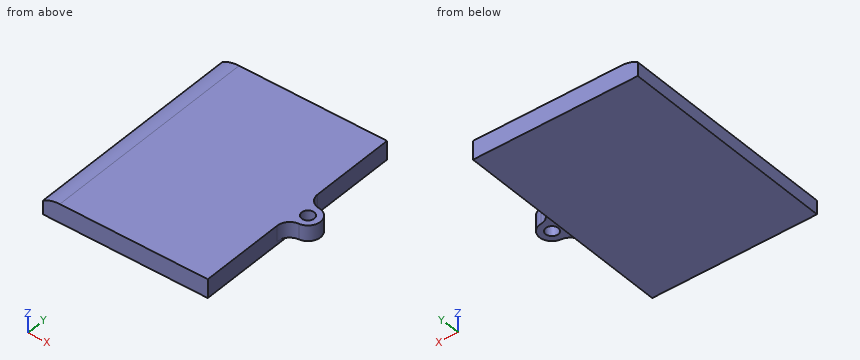
from build123d import *

# Parameters (mm, degrees)
BOSS_EXTRUDE1_DEPTH = 35.4
SKETCH2_W           = 28.62824493
SKETCH2_H           = 44.507069041
CUT_EXTRUDE1_DEPTH  = 36
SKETCH3_W           = 27
SKETCH3_H           = 2
CUT_EXTRUDE2_DEPTH  = 39.528041736
SKETCH4_W           = 4.666859097
SKETCH4_H           = 39.875061907
SKETCH4_W_2         = 6.439084071
SKETCH4_H_2         = 41.174693554
CUT_EXTRUDE3_DEPTH  = 39.563713514
SKETCH5_R           = 1
BOSS_EXTRUDE2_DEPTH = 2.5
FILLET1_R           = 2


with BuildPart() as part:
    # Sketch1 → Boss-Extrude1 (new body)
    with BuildSketch(Plane(origin=(0, 0, 0), x_dir=(1, 0, 0), z_dir=(0, 1, 0))):
        with BuildLine():
            Line((-17, 2.5), (-12, 2.5))
            Line((-12, 2.5), (12, 2.5))
            Line((12, 2.5), (12, -2.5))
            Line((12, -2.5), (-12, -2.5))
            ThreePointArc((-12, -2.5), (-15.535533906, -1.035533906), (-17, 2.5))
        make_face()
    extrude(amount=BOSS_EXTRUDE1_DEPTH)

    # Sketch2 → Cut-Extrude1 (cut)
    with BuildSketch(Plane(origin=(0, 0, -2.5), x_dir=(-1, 0, 0), z_dir=(0, 0, -1))):
        with Locations((29.314122465, 17.150131431)):
            Rectangle(SKETCH2_W, SKETCH2_H)
    extrude(amount=-CUT_EXTRUDE1_DEPTH, mode=Mode.SUBTRACT)

    # Sketch3 → Cut-Extrude2 (cut, through all)
    with BuildSketch(Plane(origin=(0, 35.4, 0), x_dir=(1, 0, 0), z_dir=(0, 1, 0))):
        with Locations((-1.5, 1.5)):
            Rectangle(SKETCH3_W, SKETCH3_H)
    extrude(amount=-CUT_EXTRUDE2_DEPTH, mode=Mode.SUBTRACT)

    # Sketch4 → Cut-Extrude3 (cut, through all)
    with BuildSketch(Plane(origin=(0, 0, -0.5), x_dir=(-1, 0, 0), z_dir=(0, 0, -1))):
        with Locations((-14.033429549, 18.67919463)):
            Rectangle(SKETCH4_W, SKETCH4_H)
        with Locations((17.919542036, 18.501972132)):
            Rectangle(SKETCH4_W_2, SKETCH4_H_2)
    extrude(amount=-CUT_EXTRUDE3_DEPTH, mode=Mode.SUBTRACT)

    # Sketch5 → Boss-Extrude2 (add)
    with BuildSketch(Plane.XY.offset(2.5)):
        with BuildLine():
            Line((13.4, 19.7), (11.7, 19.7))
            Line((11.7, 19.7), (11.7, 15.7))
            Line((11.7, 15.7), (13.4, 15.7))
            ThreePointArc((13.4, 15.7), (15.4, 17.7), (13.4, 19.7))
        make_face()
        with Locations((13.4, 17.7)):
            Circle(SKETCH5_R, mode=Mode.SUBTRACT)
    extrude(amount=-BOSS_EXTRUDE2_DEPTH)

    # Fillet1
    # the kernel refuses this fillet: 2 mm, written as the material it adds along each edge
    with BuildSketch(Plane(origin=(11.7, 15.7, 2.5), x_dir=(0, -1, 0), z_dir=(0, 0, -1))) as fillet1_piece_1:
        with BuildLine():
            CenterArc((1.988734135, -2), FILLET1_R, 90, 85.698777695)
            Line((-0.005632932, -1.85), (-0.205069639, -1.835))
            ThreePointArc((-0.205069639, -1.835), (-0.2, -1.7), (-0.2, 0))
            Line((-0.2, 0), (0, 0.2))
            Line((0, 0.2), (1.988734135, 0.2))
            Line((1.988734135, 0.2), (1.988734135, 0))
        make_face()
    extrude(amount=2.5)
    with BuildSketch(Plane(origin=(11.7, 19.7, 2.5), x_dir=(0, 1, 0), z_dir=(0, 0, -1))) as fillet1_piece_2:
        with BuildLine():
            CenterArc((1.988734135, 2), FILLET1_R, 184.301222305, 85.698777695)
            Line((-0.005632932, 1.85), (-0.205069639, 1.835))
            ThreePointArc((-0.205069639, 1.835), (-0.2, 1.7), (-0.2, 0))
            Line((-0.2, 0), (0, -0.2))
            Line((0, -0.2), (1.988734135, -0.2))
            Line((1.988734135, -0.2), (1.988734135, 0))
        make_face()
    extrude(amount=2.5)


solid = part.part
For this review, take the finished solid that the model builds, in its own axes (mm). Give positions to 0.01 mm unless a question says otherwise; leave off trailing zeros. Loops run counter-clockwise (first coordinate to the right, second up) from the corner with the lowest first, then second, coordinate; pieces in that order, holes last. Notation, with made-up numbers: (66, -21) - (117, -21) arc R21 cw to (117, -3) - close; hole circle Ø4 at (-14.5, 52.25). An arc over 180 degrees is marked (long way). Write each question's results on one line, items separated by ' | '.
(1) For pin 1 Ø1.5 at (y, z) = (22, 1.5) entering from +X; pin 2 Ø1.5 at (x, z) = (-11, 0.5) entering from -Y; pin 3 Ø1.8 at (x, y) = (13.4, 17.7) entering from +Z (3 decimals); pin 4 Ø3 at (x, y) = (14, 18.5) entering from -Z, all flat-tipped, find the tip position at first contact; note any pin that passes through.
Conclusion:
pin 1: x = 11.75 | pin 2: y = 0 | pin 3: through | pin 4: z = 0
(2) Take a section at A-A (y = 17.7). Give the boundary of the cut face in (x, z), then the cut area to 3 significant figures.
Conclusion:
outline: (-14.7, -0.5) - (11.7, -0.5) - (11.7, 0) - (12.4, 0) - (12.4, 2.5) - (-12, 2.5) arc R5 ccw to (-14.7, 1.71) - close; (14.4, 0) - (15.4, 0) - (15.4, 2.5) - (14.4, 2.5) - close | area: 82.8 mm^2
(3) Take a section at C-C (y = 23). Give the boundary of the cut face in (x, z), then the cut area to 3 significant figures.
Conclusion:
outline: (-14.7, -0.5) - (11.7, -0.5) - (11.7, 2.5) - (-12, 2.5) arc R5 ccw to (-14.7, 1.71) - close | area: 78.5 mm^2
(4) Take a section at B-B (z = 0.65). Give the boundary of the cut face in (x, y), then the cut area to 3 significant figures.
Conclusion:
outline: (-14.7, 0) - (11.7, 0) - (11.7, 13.71) arc R2 cw to (13.55, 15.71) arc R2 ccw to (13.55, 19.69) arc R2 cw to (11.7, 21.69) - (11.7, 35.4) - (-14.7, 35.4) - close; hole circle Ø2 at (13.4, 17.7) | area: 946 mm^2
(5) For line 1 along X through (y, z) = (27.5, 1.65); line 2 along Y through (x, z) = (13.4, 1.9); line 3 along Y through (x, z) = (12.5, 2.2), list the stretches that pass through material, from the lowest coordinate up.
Conclusion:
line 1: -14.7 to 11.7 | line 2: 15.69 to 16.7, 18.7 to 19.71 | line 3: 15.31 to 17.26, 18.14 to 20.09
